```python
from build123d import *

# Parameters (mm, degrees)
SKETCH3_W           = 30
SKETCH3_H           = 30
BOSS_EXTRUDE1_DEPTH = 30
SKETCH4_R           = 10
BOSS_EXTRUDE2_DEPTH = 40


with BuildPart() as part:
    # Sketch1 → Revolve1 (revolve)
    with BuildSketch(Plane.XY):
        with BuildLine():
            Line((0, 74.602122016), (0, -75.397877984))
            Line((0, -75.397877984), (80, -75.397877984))
            Line((80, -75.397877984), (80, -7.360742706))
            ThreePointArc((80, -7.360742706), (74, -1.360742706), (80, 4.639257294))
            Line((80, 4.639257294), (80, 20.050397878))
            ThreePointArc((80, 20.050397878), (72, 28.050397878), (80, 36.050397878))
            Line((80, 36.050397878), (80, 74.602122016))
            Line((80, 74.602122016), (0, 74.602122016))
        make_face()
    revolve(axis=Axis((0, 74.602122016, 0), (0, -1, 0)))

    # Sketch3 → Boss-Extrude1 (add)
    with BuildSketch(Plane.XZ.offset(75.397877984)):
        with Locations((0, -35)):
            Rectangle(SKETCH3_W, SKETCH3_H)
        with Locations((0, 35)):
            Rectangle(SKETCH3_W, SKETCH3_H)
    extrude(amount=BOSS_EXTRUDE1_DEPTH)

    # Sketch4 → Boss-Extrude2 (add)
    with BuildSketch(Plane(origin=(0, 0, 20), x_dir=(-1, 0, 0), z_dir=(0, 0, -1))):
        with Locations((0, -90.397877984)):
            Circle(SKETCH4_R)
    extrude(amount=BOSS_EXTRUDE2_DEPTH)


solid = part.part
```
Geometry: final body of the model. Coordinates: model frame, mm. A direction names the side the tool comes from. Coordinates: 2 decimals unless noted, no trailing zeros. Order: outer loops, then holes, each group sorted by start corner. A loop starts at its lowest first (then second) coordinate and runs counter-clockwise, first axis right, second up. Notation, with made-up numbers: (54, 33.5) - (75, 33.5) arc R32 cw to (75, 59.5) - close; hole circle Ø2 at (-33.5, 60.25). An arc over 180 degrees is marked (long way). Write each question's results on one line, items separated by ' | '.
1) Line query: line 1 (Y direction, x = 73, z = -25); line 2 (Y direction, x = -9, z = 6); line 3 (Y direction, x = 55.5, z = 11). Output: solid intervals per line, ascending. Write a range as from..to.
Results list:
line 1: -75.4..-6.65, 3.93..20.57, 35.53..74.6 | line 2: -94.76..-86.04, -75.4..74.6 | line 3: -75.4..74.6
2) Set-up query: faces 4 (the flat face through (0, -90, 50)), 5 (the flat face through (0, -80, -20)), 6 (the flat face through (-15, -90, -35)), 7 (the flat face through (0, -90, -50)), 8 (the flat face through (15, -90, 35)). Return all of +Z, -Z, +X, -X, +Y, -Y with unobstructed straight access to the full face (end or side cutting, diameter ignored); none if empty.
Results list:
face 4: +Z, +X, -X, -Y | face 5: none | face 6: +Z, -Z, -X, -Y | face 7: -Z, +X, -X, -Y | face 8: +Z, -Z, +X, -Y
3) Pull-direction query (Y, two-part tool) for faces 1 (the flat face through (0, -105.398, -35)), 2 (the flat face through (15, -90, -35)), 3 (the flat face through (0, -80, 20)); classes: pulls with the +Y half, pulls with the -Y half, needs draft (parallel to the pull), parting line crosses it, or undercut.
Results list:
face 1: pulls with the -Y half | face 2: needs draft | face 3: undercut
4) Section B-B, the plane z = 0. Return loops of the section in (x, y), plus the area to 3 significant figures.
Results list:
outline: (-80, -75.4) - (80, -75.4) - (80, -7.36) arc R6 cw to (80, 4.64) - (80, 20.05) arc R8 cw to (80, 36.05) - (80, 74.6) - (-80, 74.6) - (-80, 36.05) arc R8 cw to (-80, 20.05) - (-80, 4.64) arc R6 cw to (-80, -7.36) - close; circle Ø20 at (0, -90.4) | area: 24,000 mm^2
5) Section C-C, the plane y = -52. Return loops of the section in (x, z).
Results list:
outline: circle Ø160 at (0, 0)
6) Section A-A, the plane x = 0. Return loops of the section in (y, z), plus the area to 3 significant figures.
Results list:
outline: (-105.4, -50) - (-75.4, -50) - (-75.4, -80) - (-7.36, -80) arc R6 cw to (4.64, -80) - (20.05, -80) arc R8 cw to (36.05, -80) - (74.6, -80) - (74.6, 80) - (36.05, 80) arc R8 cw to (20.05, 80) - (4.64, 80) arc R6 cw to (-7.36, 80) - (-75.4, 80) - (-75.4, 50) - (-105.4, 50) - (-105.4, 20) - (-100.4, 20) - (-100.4, -20) - (-105.4, -20) - close; hole (-80.4, -20) - (-75.4, -20) - (-75.4, 20) - (-80.4, 20) - close | area: 26,300 mm^2
7) Pin query (flat end, axial travel): pin 1 (4 mm diameter, centred on x = -28.5, y = -3.5, fed in from +Z); pin 2 (24 mm diameter, centred on x = 1, y = -87.5, fed in from -Z); pin 3 (5 mm diameter, centred on y = -67.5, z = 18, fed in from -X). Return the tip coordinate at first contact, or that it passes through.
Results list:
pin 1: z = 70.24 | pin 2: z = -50 | pin 3: x = -78.48
8) Section D-D, the plane y = -3.5. Return loops of the section in (x, z).
Results list:
outline: circle Ø148.79 at (0, 0)
